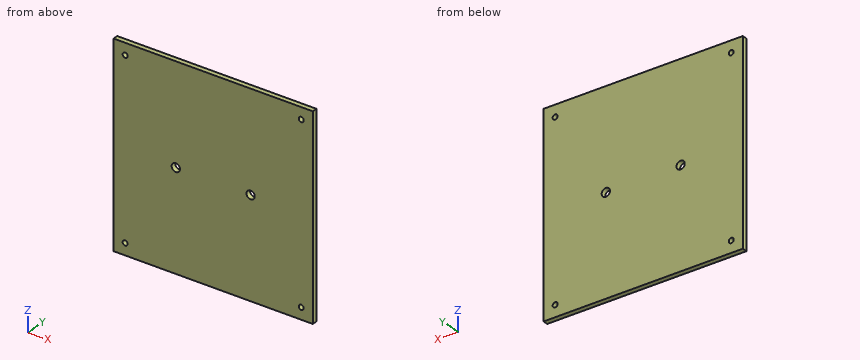
```python
from build123d import *

# Parameters (mm, degrees)
SKETCH1_W           = 120
SKETCH1_H           = 120
BOSS_EXTRUDE1_DEPTH = 3
SKETCH4_R           = 2.5
CUT_EXTRUDE2_DEPTH  = 3
SKETCH7_R           = 1.5
CUT_EXTRUDE3_DEPTH  = 3


with BuildPart() as part:
    # Sketch1 → Boss-Extrude1 (new body)
    with BuildSketch(Plane(origin=(0, 0, 0), x_dir=(1, 0, 0), z_dir=(0, 1, 0))):
        Rectangle(SKETCH1_W, SKETCH1_H)
    extrude(amount=BOSS_EXTRUDE1_DEPTH)

    # Sketch4 → Cut-Extrude2 (cut)
    with BuildSketch(Plane(origin=(0, 0, 0), x_dir=(1, 0, 0), z_dir=(0, 1, 0))):
        with Locations((-22.5, 0)):
            Circle(SKETCH4_R)
        with Locations((22.5, 0)):
            Circle(SKETCH4_R)
    extrude(amount=CUT_EXTRUDE2_DEPTH, mode=Mode.SUBTRACT)

    # Sketch7 → Cut-Extrude3 (cut)
    with BuildSketch(Plane(origin=(0, 0, 0), x_dir=(1, 0, 0), z_dir=(0, 1, 0))):
        with Locations((-53, 53)):
            Circle(SKETCH7_R)
        with Locations((53, 53)):
            Circle(SKETCH7_R)
        with Locations((-53, -53)):
            Circle(SKETCH7_R)
        with Locations((53, -53)):
            Circle(SKETCH7_R)
    extrude(amount=CUT_EXTRUDE3_DEPTH, mode=Mode.SUBTRACT)


solid = part.part
```
Check sheet for the modelled part. Datum: model origin and axes. Units: mm. Give positions to 0.01 mm unless a question says otherwise; leave off trailing zeros. Order: outer loops, then holes, each group sorted by start corner. A loop starts at its lowest first (then second) coordinate and runs counter-clockwise, first axis right, second up. Notation, with made-up numbers: M 10.5,8 L 16.5,8 A11 ccw 16.5,25 Z; hole C 78.5,-37 d3. An arc over 180 degrees is marked long. Answer in a Markdown table with one row per item.
1) Cross-section at A-A, the plane x = -53. Enter the section's corners in (y, z).
Filled sheet:
| item | result |
|---|---|
| outline | M 0,-60 L 3,-60 L 3,-54.5 L 0,-54.5 Z; M 0,-51.5 L 3,-51.5 L 3,51.5 L 0,51.5 Z; M 0,54.5 L 3,54.5 L 3,60 L 0,60 Z |
2) Cross-section at B-B, the plane z = 0. Enter the section's corners in (x, y).
Filled sheet:
| item | result |
|---|---|
| outline | M -60,0 L -25,0 L -25,3 L -60,3 Z; M -20,0 L 20,0 L 20,3 L -20,3 Z; M 25,0 L 60,0 L 60,3 L 25,3 Z |
3) Thickness scan on L1, parallel to Z at x = -53, y = 0.9; L2, parallel to X at y = 1, z = 0. Record the ranges inside material, lowest first. Write a range as [from, to].
Filled sheet:
| item | result |
|---|---|
| L1 | z = [-60, -54.5], [-51.5, 51.5], [54.5, 60] |
| L2 | x = [-60, -25], [-20, 20], [25, 60] |
4) Gauge pin test, flat end, axial feed: P1, Ø3, axis at x = -22.5, z = 0, coming from the +Y side (3 decimals). Record the tip position at first contact, or that the pin passes through.
Filled sheet:
| item | result |
|---|---|
| P1 | passes through |
5) Cross-section at C-C, the plane x = 22.5. Enter the section's corners in (y, z).
Filled sheet:
| item | result |
|---|---|
| outline | M 0,-60 L 3,-60 L 3,-2.5 L 0,-2.5 Z; M 0,2.5 L 3,2.5 L 3,60 L 0,60 Z |
